```python
from build123d import *

# Parameters (mm, degrees)
F1_DEPTH = 76.2
F2_R     = 12.7
F3_DEPTH = 20.52468


with BuildPart() as f1:
    # F0 (on Front) → F1 (new body)
    with BuildSketch(Plane.XZ):
        with BuildLine():
            ThreePointArc((207.101302, 0), (174.548609, 28.020886), (133.35, 15.875))
            Line((133.35, 15.875), (-133.35, 15.875))
            ThreePointArc((-133.35, 15.875), (-174.548609, 28.020886), (-207.101302, 0))
            Line((-207.101302, 0), (-194.799406, -4.64968))
            ThreePointArc((-194.799406, -4.64968), (-165.1, 15.875), (-135.400594, -4.64968))
            Line((-135.400594, -4.64968), (135.400594, -4.64968))
            ThreePointArc((135.400594, -4.64968), (165.1, 15.875), (194.799406, -4.64968))
            Line((194.799406, -4.64968), (207.101302, 0))
        make_face()
    extrude(amount=F1_DEPTH)

    # F2 (on face) → F3 (cut, through all)
    with BuildSketch(Plane.XY.offset(15.875)):
        with Locations((0, -38.1)):
            Circle(F2_R)
    extrude(amount=-F3_DEPTH, mode=Mode.SUBTRACT)


solid = f1.part
```
Model file for the job. Use its own axes, mm. A direction names the side the tool comes from. Give positions to 0.01 mm unless a question says otherwise; leave off trailing zeros. Write each loop counter-clockwise with the first axis right and the second up, starting at its lowest first coordinate (ties: lowest second). Pieces come first, ordered by that corner, then holes. Notation, with made-up numbers: M 73,-1.75 L 88,-1.75 A11 cw 88,18.25 Z; hole C -32.75,-24 d4. An arc over 180 degrees is marked long. Use a Markdown table: item, result.
1) Drill centre lines: line 1 (Y direction, x = 0, z = 3.25); line 2 (X direction, y = -38, z = 2); line 3 (X direction, y = -40.5, z = 11). Where is each one in solid material? Low to high. Write a range as from..to.
Responses:
| item | result |
|---|---|
| line 1 | y = -76.2..-50.8, -25.4..0 |
| line 2 | x = -206.29..-191.34, -138.86..-12.7, 12.7..138.86, 191.34..206.29 |
| line 3 | x = -201.07..-182.01, -148.19..-12.47, 12.47..148.19, 182.01..201.07 |
2) Tool access for faces 1 (the flat face through (2, -54, 15.875)), 2 (the cylindrical face through (-2.75, -50.5, 5.76)): list every direction of +Z, -Z, +X, -X, +Y, -Y with a clear straight run to the whole face (end or side of a thin tool).
Responses:
| item | result |
|---|---|
| face 1 | +Z, +Y, -Y |
| face 2 | +Z, -Z |
3) Cut at D-D (x = 176). List the corners of the cut face in (y, z).
Responses:
| item | result |
|---|---|
| outline | M -76.2,13.95 L 0,13.95 L 0,27.68 L -76.2,27.68 Z |
4) Cut at C-C (x = 115.5). List the corners of the cut face in (y, z) (3 decimals).
Responses:
| item | result |
|---|---|
| outline | M -76.2,-4.65 L 0,-4.65 L 0,15.875 L -76.2,15.875 Z |
5) Cut at A-A (x = 0). List the corners of the cut face in (y, z) (3 decimals), and give its area (3 significant figures).
Responses:
| item | result |
|---|---|
| outline | M -76.2,-4.65 L -50.8,-4.65 L -50.8,15.875 L -76.2,15.875 Z; M -25.4,-4.65 L 0,-4.65 L 0,15.875 L -25.4,15.875 Z |
| area | 1,040 mm2 |
6) Pin check, flat tips, straight feed: pin 1 (2 mm diameter, centred on y = -66.5, z = 7.5, fed in from -X); pin 2 (1 mm diameter, centred on x = -53.5, z = 3, fed in from +Y); pin 3 (5 mm diameter, centred on y = -63.5, z = 15, fed in from +X); pin 4 (6 mm diameter, centred on y = -28, z = 1.5, fed in from -X). Stop position of each tip, or through.
Responses:
| item | result |
|---|---|
| pin 1 | stops at x = -204.03 |
| pin 2 | stops at y = 0 |
| pin 3 | stops at x = 199.9 |
| pin 4 | stops at x = -207.1 |
7) Cut at B-B (y = -38.1). List the corners of the cut face in (x, z) (3 decimals), and give its area (3 significant figures).
Responses:
| item | result |
|---|---|
| outline | M -207.101,0 L -194.799,-4.65 A31.75 cw -135.401,-4.65 L -12.7,-4.65 L -12.7,15.875 L -133.35,15.875 A44.901 ccw Z; M 12.7,-4.65 L 135.401,-4.65 A31.75 cw 194.799,-4.65 L 207.101,0 A44.901 ccw 133.35,15.875 L 12.7,15.875 Z |
| area | 7,160 mm2 |
8) Pull direction X, two halves, no side cores. Call faces 3 (the flat face through (-3, 0, 9)), 4 (the cylindrical face through (-173.93, -37.57, 28.15)), 5 (the flat face through (-201.04, -37.57, -2.29)): +X half, -X half, draft (parallel to the pull), parting line (faces both ways), or undercut.
Responses:
| item | result |
|---|---|
| face 3 | draft |
| face 4 | undercut |
| face 5 | -X half |
